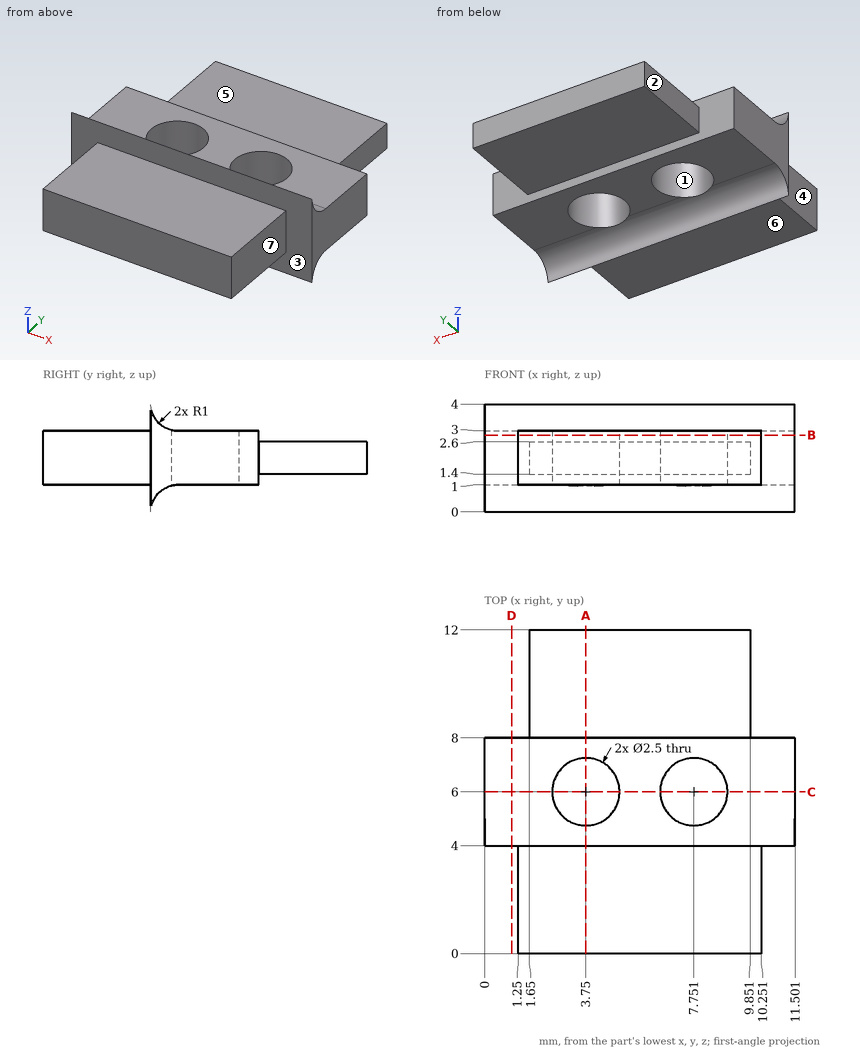
Print and shaded views of the part. All mm, measured from the part's lowest x, y and z. A direction names the side the tool comes from. Round coordinates to 2 decimals unless told otherwise and drop trailing zeros. Write each loop counter-clockwise with the first axis right and the second up, starting at its lowest first coordinate (ties: lowest second). Pieces come first, ordered by that corner, then holes. Notation, with made-up numbers: (79.5, 81) -> (132.5, 81) arc R28 ccw to (132.5, 114) -> close; hole circle Ø11 at (36.5, 35). An arc over 180 degrees is marked (long way). Answer in a Markdown table with one row per item. Add a question column.
Item 1: Saw through at C-C, the plane y = 6. Write the cut outline in (x, z), then the cut area to 3 significant figures.
Item 2: Mould opens along X. For the marked faces 1, 2 and 3 say: pulls with the +X half, pulls with the -X half, needs draft (parallel to the pull), parting line crosses it, or undercut.
Item 3: Which spindle directions (+Z, -Z, +X, -X, +Y, -Y) get a long thin tool onto all of the face, cutting with end or side? Do the marked faces 4, 5, 6 and 7. Say none if no direction does.
Item 4: Saw through at A-A, the plane x = 3.75. Write the cut outline in (y, z).
Item 5: Drill centre lines: line 1 (X direction, y = 6, z = 2.35); line 2 (X direction, y = 6.75, z = 2.85); line 3 (Y direction, x = 3.75, z = 1.6). Where is each one in solid material? Low to high. Write a range as from..to.
Item 6: Drop flat-ended pins along their axis: pin 1 Ø1 at (y, z) = (11, 2) entering from +X; pin 2 Ø4.5 at (x, y) = (4, 1) entering from -Z; pin 3 Ø1.6 at (y, z) = (2.5, 2.5) entering from -X. Give the stop position or say it passes through.
Item 7: Saw through at B-B, the plane z = 2.85. Write the cut outline in (x, y), then the cut area to 3 significant figures.
Item 8: Saw through at D-D, the plane x = 1. Write the cut outline in (y, z).
Findings below:
| question | item | result |
|---|---|---|
| 1 | outline | (0, 1) -> (2.5, 1) -> (2.5, 3) -> (0, 3) -> close; (5, 1) -> (6.5, 1) -> (6.5, 3) -> (5, 3) -> close; (9, 1) -> (11.5, 1) -> (11.5, 3) -> (9, 3) -> close |
| 1 | area | 13.0 mm^2 |
| 2 | face 1 | undercut |
| 2 | face 2 | pulls with the -X half |
| 2 | face 3 | needs draft |
| 3 | face 4 | +Z, -Z, -X, -Y |
| 3 | face 5 | +Z, +X, -X, +Y |
| 3 | face 6 | -Z, +X, -X, -Y |
| 3 | face 7 | +Z, -Z, +X, -Y |
| 4 | outline | (0, 1) -> (4, 1) -> (4, 0) arc R1 cw to (4.75, 0.97) -> (4.75, 3.03) arc R1 cw to (4, 4) -> (4, 3) -> (0, 3) -> close; (7.25, 1) -> (8, 1) -> (8, 1.4) -> (12, 1.4) -> (12, 2.6) -> (8, 2.6) -> (8, 3) -> (7.25, 3) -> close |
| 5 | line 1 | x = 0..2.5, 5..6.5, 9..11.5 |
| 5 | line 2 | x = 0..2.75, 4.75..6.75, 8.75..11.5 |
| 5 | line 3 | y = 0..4.75, 7.25..12 |
| 6 | pin 1 | stops at x = 9.85 |
| 6 | pin 2 | stops at z = 1 |
| 6 | pin 3 | stops at x = 1.25 |
| 7 | outline | (0, 4) -> (1.25, 4) -> (1.25, 0) -> (10.25, 0) -> (10.25, 4) -> (11.5, 4) -> (11.5, 8) -> (0, 8) -> close; hole circle Ø2.5 at (3.75, 6); hole circle Ø2.5 at (7.75, 6) |
| 7 | area | 72.2 mm^2 |
| 8 | outline | (4, 0) arc R1 cw to (5, 1) -> (8, 1) -> (8, 3) -> (5, 3) arc R1 cw to (4, 4) -> close |
